Drawing for the job (mm, zero at the part's lowest x, y, z). A direction names the side the tool comes from. Coordinates: 2 decimals unless noted, no trailing zeros. Order: outer loops, then holes, each group sorted by start corner. A loop starts at its lowest first (then second) coordinate and runs counter-clockwise, first axis right, second up. Notation, with made-up numbers: (-10.75, 27.5) -> (42.25, 27.5) arc R18 cw to (42.25, 54.5) -> close; hole circle Ø7 at (-7.75, -21.75). An arc over 180 degrees is marked (long way). Write each question's results on one line, items separated by ' | '.
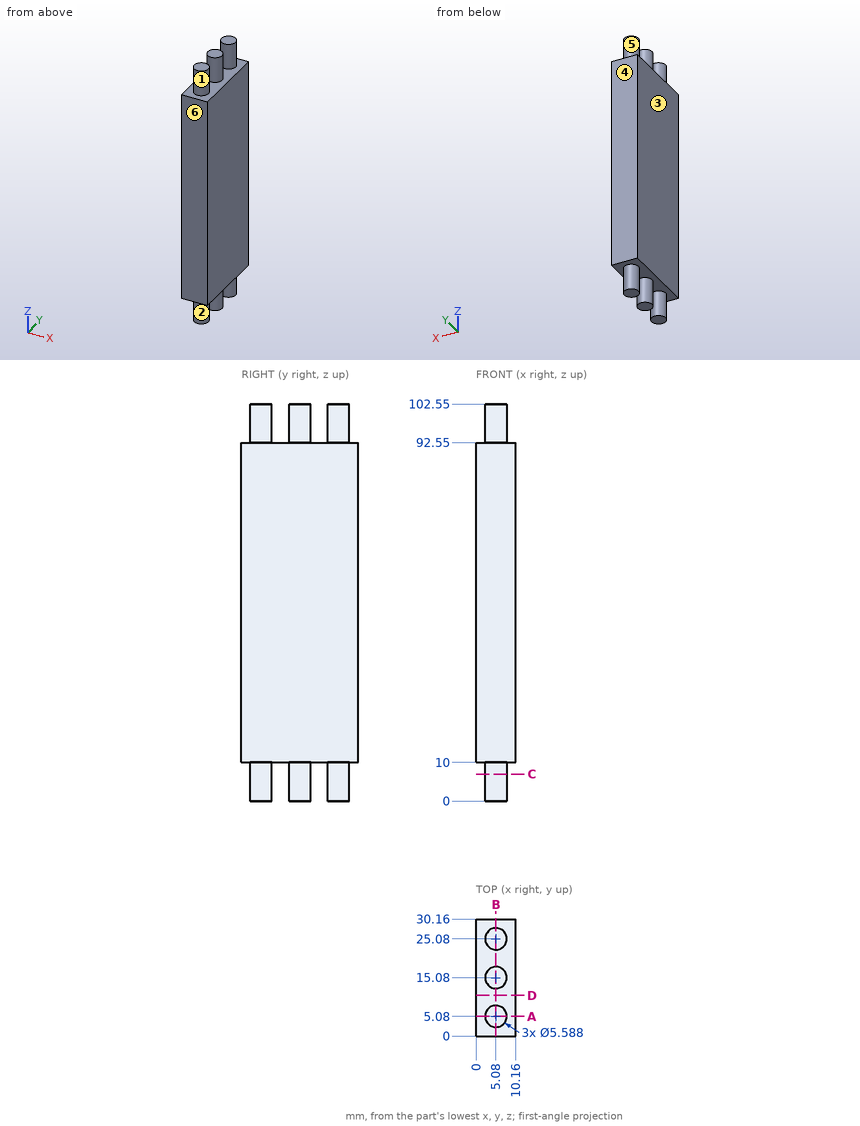
Item 1: Tool access for the marked faces 1, 2 and 3: list every direction of +Z, -Z, +X, -X, +Y, -Y with a clear straight run to the whole face (end or side of a thin tool).
Answer:
face 1: +Z | face 2: -Z | face 3: +Z, -Z, -X, +Y, -Y
Item 2: Slice it at B-B, the plane x = 5.08. List the corners of the cut face in (y, z).
Answer:
outline: (0, 10) -> (2.29, 10) -> (2.29, 0) -> (7.87, 0) -> (7.87, 10) -> (12.29, 10) -> (12.29, 0) -> (17.87, 0) -> (17.87, 10) -> (22.29, 10) -> (22.29, 0) -> (27.87, 0) -> (27.87, 10) -> (30.16, 10) -> (30.16, 92.55) -> (27.87, 92.55) -> (27.87, 102.55) -> (22.29, 102.55) -> (22.29, 92.55) -> (17.87, 92.55) -> (17.87, 102.55) -> (12.29, 102.55) -> (12.29, 92.55) -> (7.87, 92.55) -> (7.87, 102.55) -> (2.29, 102.55) -> (2.29, 92.55) -> (0, 92.55) -> close
Item 3: Slice it at D-D, the plane y = 10.5. List the corners of the cut face in (x, z), and give its area (3 significant figures).
Answer:
outline: (0, 10) -> (10.16, 10) -> (10.16, 92.55) -> (0, 92.55) -> close | area: 839 mm^2
Item 4: Slice it at A-A, the plane y = 5.08. List the corners of the cut face in (x, z), and give its area (3 significant figures).
Answer:
outline: (0, 10) -> (2.29, 10) -> (2.29, 0) -> (7.87, 0) -> (7.87, 10) -> (10.16, 10) -> (10.16, 92.55) -> (7.87, 92.55) -> (7.87, 102.55) -> (2.29, 102.55) -> (2.29, 92.55) -> (0, 92.55) -> close | area: 950 mm^2
Item 5: Drill centre lines: line 1 (Y direction, x = 6.25, z = 4.5); line 2 (Z direction, x = 4.5, y = 2); line 3 (X direction, y = 13.5, z = 96). Where is each one in solid material? Low to high. Write a range as from..to.
Answer:
line 1: y = 2.54..7.62, 12.54..17.62, 22.54..27.62 | line 2: z = 10..92.55 | line 3: x = 2.78..7.38
Item 6: Pull direction Y, two halves, no side cores. Call the marked faces 4, 5 and 6: released by +Y, released by -Y, zero draft, split by the parting line, or undercut.
Answer:
face 4: released by +Y | face 5: undercut | face 6: released by -Y
Item 7: Slice it at C-C, the plane z = 7. List the corners of the cut face in (x, y).
Answer:
outline: circle Ø5.59 at (5.08, 5.08); circle Ø5.59 at (5.08, 15.08); circle Ø5.59 at (5.08, 25.08)
